Geometry: final body of the model. Coordinates: model frame, mm. A direction names the side the tool comes from. Round coordinates to 2 decimals unless told otherwise and drop trailing zeros. Loops run counter-clockwise (first coordinate to the right, second up) from the corner with the lowest first, then second, coordinate; pieces in that order, holes last. Notation, with made-up numbers: (-28, 16.5) -> (-7, 16.5) arc R25 ccw to (-7, 33.5) -> close; hole circle Ø1 at (81.5, 80). An arc over 180 degrees is marked (long way). Answer in a Markdown table with one row per item.
```python
from build123d import *

# Parameters (mm, degrees)
F0_R     = 10.9
F1_DEPTH = 14.732


with BuildPart() as f1:
    # F0 (on Front) → F1 (new body)
    with BuildSketch(Plane.XZ):
        Polygon((10.065964, 50.761367), (6.456376, 49.49288), (2.45947, 46.763286), (0, 44.131174), (-2.024869, 39.841811), (-2.999724, 35.942386), (-2.024869, 31.165595), (0, 25.413946), (0, 22.001951), (1.09467, 17.517616), (1.09467, 8.451459), (1.09467, 5.13695), (0, 1.140108), (0, -2.856889), (-1.732659, -7.536301), (-2.610176, -10.363446), (-2.610176, -13.19059), (-2.610176, -16.895124), (-0.953385, -21.574536), (0, -25.181582), (7.722604, -30.933358), (18.641215, -30.933358), (18.641215, -31.32331), (24.880612, -27.228824), (28.097883, -23.329314), (29.657858, -19.527293), (29.657858, -16.895124), (29.657858, -12.3132), (28.097883, -7.536301), (27.026469, -2.076987), (25.856924, 5.13695), (25.856924, 12.156223), (25.856924, 19.955242), (28.097883, 27.364309), (29.657858, 31.848747), (29.657858, 37.015595), (28.097883, 41.792495), (23.031681, 47.349298), (18.641215, 50.273932), (16.20773, 51.63876), (13.478043, 51.63876), align=None)
        Polygon((22.879082, -19.204851), (17.902447, -27.764871), (8.000935, -27.734988), (3.076058, -19.145086), (8.052694, -10.585066), (17.954206, -10.614949), align=None, mode=Mode.SUBTRACT)
        Polygon((17.902447, 44.667789), (22.879082, 36.10777), (17.954206, 27.517867), (8.052694, 27.487984), (3.076058, 36.048004), (8.000935, 44.637906), align=None, mode=Mode.SUBTRACT)
        with Locations((13.388105, 11.897694)):
            Circle(F0_R, mode=Mode.SUBTRACT)
    extrude(amount=F1_DEPTH)


solid = f1.part
```
Item 1: Set-up query: faces 5 (the flat face through (4.49, -7.26, 48.15)), 6 (the flat face through (26.962, -7.263, 23.608)), 7 (the flat face through (20.45, -7.26, 31.87)), 8 (the flat face through (-1.793, -7.263, -19.202)), 9 (the flat face through (0.555, -7.263, 3.167)). Return all of +Z, -Z, +X, -X, +Y, -Y with unobstructed straight access to the full face (end or side cutting, diameter ignored); none if empty.
Ans:
| item | result |
|---|---|
| face 5 | +Z, -X, +Y, -Y |
| face 6 | +X, +Y, -Y |
| face 7 | +Y, -Y |
| face 8 | -Z, -X, +Y, -Y |
| face 9 | -X, +Y, -Y |
Item 2: First-contact query: P1, Ø2, axis at x = 8, y = -4.5, coming from the +Z side; P2, Ø2, axis at y = -8, z = 10.5, coming from the -X side; P3, Ø2, axis at y = -10.5, z = -1, coming from the -X side; P4, Ø19.5, axis at x = 13.39, z = 11.9, coming from the +Y side. Flat tips, straight axial feed; report the tip coordinate or a pass-through.
Ans:
| item | result |
|---|---|
| P1 | z = 50.39 |
| P2 | x = 1.09 |
| P3 | x = 0 |
| P4 | through |
Item 3: Section query A-A, the plane z = 28.5. Output: boundary loops of the cut face in (x, y).
Ans:
| item | result |
|---|---|
| outline | (-1.09, -14.73) -> (7.46, -14.73) -> (7.46, 0) -> (-1.09, 0) -> close; (18.52, -14.73) -> (28.49, -14.73) -> (28.49, 0) -> (18.52, 0) -> close |
Item 4: Section query C-C, the plane z = 10.5. Output: boundary loops of the cut face in (x, y).
Ans:
| item | result |
|---|---|
| outline | (1.09, -14.73) -> (2.58, -14.73) -> (2.58, 0) -> (1.09, 0) -> close; (24.2, -14.73) -> (25.86, -14.73) -> (25.86, 0) -> (24.2, 0) -> close |
Item 5: Section query D-D, the plane x = 5. Output: boundary loops of the cut face in (y, z).
Ans:
| item | result |
|---|---|
| outline | (-14.73, -28.91) -> (0, -28.91) -> (0, -22.5) -> (-14.73, -22.5) -> close; (-14.73, -15.84) -> (0, -15.84) -> (0, 4.94) -> (-14.73, 4.94) -> close; (-14.73, 18.86) -> (0, 18.86) -> (0, 32.74) -> (-14.73, 32.74) -> close; (-14.73, 39.4) -> (0, 39.4) -> (0, 48.5) -> (-14.73, 48.5) -> close |
Item 6: Mould query, pull axis X, two halves, no side actions, for faces 1 (the flat face through (15, -7, 51.639)), 2 (the flat face through (25.6, -7.26, 44.53)), 3 (the flat face through (20.356, -7.263, 40.448)), 4 (the flat face through (-1.027, -7.263, 28.33)). Classes: released by +X, released by -X, zero draft, split by the parting line, or undercut.
Ans:
| item | result |
|---|---|
| face 1 | zero draft |
| face 2 | released by +X |
| face 3 | undercut |
| face 4 | released by -X |
Item 7: Section query B-B, the plane x = 11. Output: boundary loops of the cut face in (y, z), and give its area (3 significant figures).
Ans:
| item | result |
|---|---|
| outline | (-14.73, -30.93) -> (0, -30.93) -> (0, -27.74) -> (-14.73, -27.74) -> close; (-14.73, -10.59) -> (0, -10.59) -> (0, 1.26) -> (-14.73, 1.26) -> close; (-14.73, 22.53) -> (0, 22.53) -> (0, 27.5) -> (-14.73, 27.5) -> close; (-14.73, 44.65) -> (0, 44.65) -> (0, 51) -> (-14.73, 51) -> close |
| area | 388 mm2 |
Item 8: Ray query, L1, parallel to Z at x = 14, y = -4.25; L2, parallel to Z at x = 12.5, y = -9; L3, parallel to X at y = -13.5, z = 10. Return the intervals inside material, ascending.
Ans:
| item | result |
|---|---|
| L1 | -30.93 to -27.75, -10.6 to 1.01, 22.78 to 27.51, 44.66 to 51.64 |
| L2 | -30.93 to -27.75, -10.6 to 1.03, 22.76 to 27.5, 44.65 to 51.39 |
| L3 | 1.09 to 2.65, 24.12 to 25.86 |
